Geometry: see drawing. Coordinates: mm, zero at the bounding-box minimum. A direction names the side the tool comes from. Give positions to 0.01 mm unless a question says otherwise; leave off trailing zeros. Write each loop counter-clockwise with the first axis right and the second up, starting at its lowest first coordinate (ties: lowest second). Pieces come first, ordered by that corner, then holes. Notation, with made-up numbers: (-18.5, 21) - (29.5, 21) arc R14 cw to (29.5, 48) - close; hole circle Ø7 at (-19.5, -4.5). An arc over 180 degrees is marked (long way). Return JSON: item names as keys, results as strings.
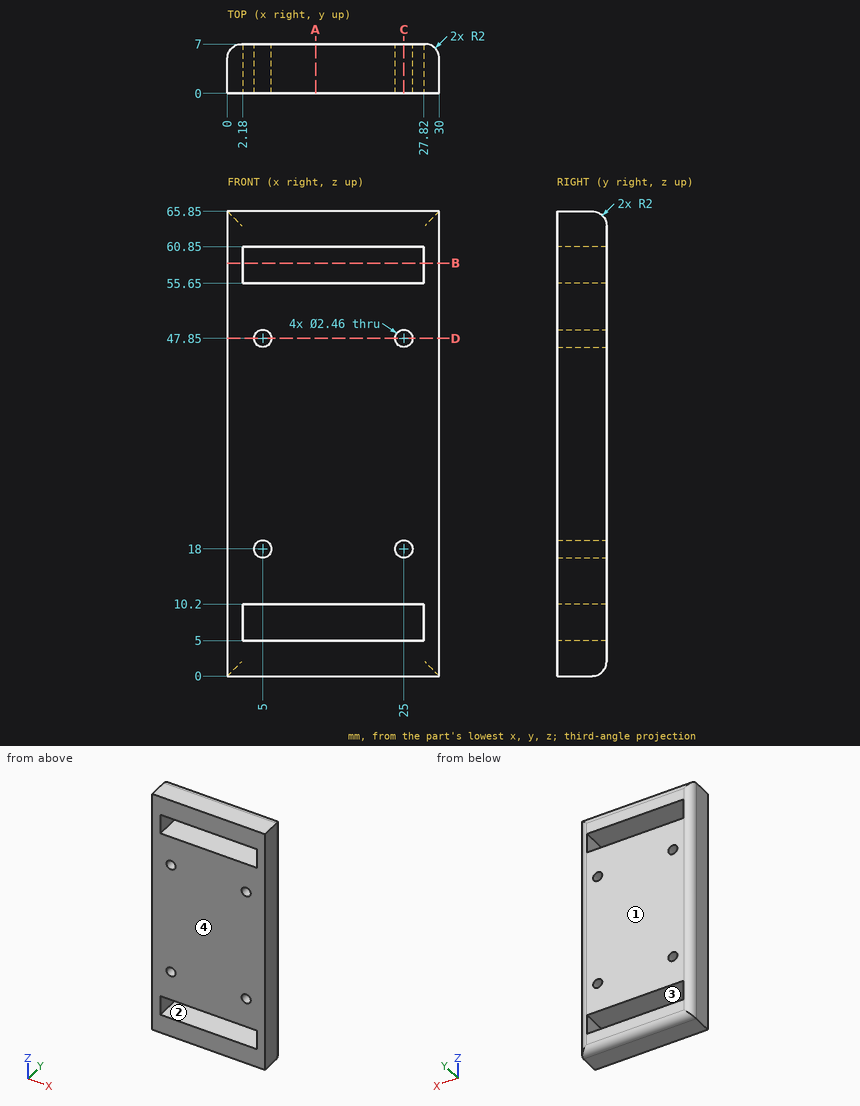
Q1. Section query B-B, the plane z = 58.5. Return the cut outline in (x, y).
Answer key:
{"outline": "(0, 0) - (2.18, 0) - (2.18, 7) - (2, 7) arc R2 ccw to (0, 5) - close; (27.82, 0) - (30, 0) - (30, 5) arc R2 ccw to (28, 7) - (27.82, 7) - close"}
Q2. Section query D-D, the plane z = 47.85. Return the cut outline in (x, y), plus the area to 3 significant figures.
Answer key:
{"outline": "(0, 0) - (3.77, 0) - (3.77, 7) - (2, 7) arc R2 ccw to (0, 5) - close; (6.23, 0) - (23.77, 0) - (23.77, 7) - (6.23, 7) - close; (26.23, 0) - (30, 0) - (30, 5) arc R2 ccw to (28, 7) - (26.23, 7) - close", "area": "174 mm^2"}
Q3. Set-up query: the marked faces 3 and 4. Return all of +Z, -Z, +X, -X, +Y, -Y with unobstructed straight access to the full face (end or side cutting, diameter ignored); none if empty.
Answer key:
{"face 3": "+Y, -Y", "face 4": "+Z, -Z, +X, -X, -Y"}
Q4. Section query A-A, the plane x = 12.5. Return the cut outline in (y, z), plus the area to 3 significant figures.
Answer key:
{"outline": "(0, 0) - (5, 0) arc R2 ccw to (7, 2) - (7, 5) - (0, 5) - close; (0, 10.2) - (7, 10.2) - (7, 55.65) - (0, 55.65) - close; (0, 60.85) - (7, 60.85) - (7, 63.85) arc R2 ccw to (5, 65.85) - (0, 65.85) - close", "area": "386 mm^2"}
Q5. Mould query, pull axis Z, two halves, no side actions, for the marked faces 1 and 2. Classes: pulls with the +Z half, pulls with the -Z half, needs draft (parallel to the pull), parting line crosses it, or undercut.
Answer key:
{"face 1": "needs draft", "face 2": "undercut"}
Q6. Section query C-C, the plane x = 25. Return the cut outline in (y, z), plus the area to 3 significant figures.
Answer key:
{"outline": "(0, 0) - (5, 0) arc R2 ccw to (7, 2) - (7, 5) - (0, 5) - close; (0, 10.2) - (7, 10.2) - (7, 16.77) - (0, 16.77) - close; (0, 19.23) - (7, 19.23) - (7, 46.62) - (0, 46.62) - close; (0, 49.08) - (7, 49.08) - (7, 55.65) - (0, 55.65) - close; (0, 60.85) - (7, 60.85) - (7, 63.85) arc R2 ccw to (5, 65.85) - (0, 65.85) - close", "area": "352 mm^2"}
Q7. Material intervals for probe 1 along X at (y, z) = (4.25, 47.85); probe 2 along Z at (x, y) = (5, 3.5); probe 3 along Z at (x, y) = (12.75, 1.5), sorted ascending. Write a range as [from, to].
Answer key:
{"probe 1": "x = [0, 3.77], [6.23, 23.77], [26.23, 30]", "probe 2": "z = [0, 5], [10.2, 16.77], [19.23, 46.62], [49.08, 55.65], [60.85, 65.85]", "probe 3": "z = [0, 5], [10.2, 55.65], [60.85, 65.85]"}
